```python
from build123d import *

# Parameters (mm, degrees)
SKETCH1_W           = 50.8
SKETCH1_H           = 25.4
BOSS_EXTRUDE1_DEPTH = 5.08
FILLET2_RADIUS      = 2.54
FILLET2_LENGTH      = 25.4
FILLET3_RADIUS      = 2.54
FILLET3_LENGTH      = 25.4
SKETCH2_R           = 2.54
BOSS_EXTRUDE2_DEPTH = 12.7
BOSS_EXTRUDE3_START = 12.7
SKETCH3_R           = 2.54
BOSS_EXTRUDE3_DEPTH = 12.7
SKETCH4_W           = 52.876932696
SKETCH4_H           = 9.818783706
CUT_EXTRUDE1_DEPTH  = 12.7


with BuildPart() as part:
    # Sketch1 → Boss-Extrude1 (new body)
    with BuildSketch(Plane(origin=(0, 0, 0), x_dir=(1, 0, 0), z_dir=(0, 1, 0))):
        Rectangle(SKETCH1_W, SKETCH1_H)
    extrude(amount=BOSS_EXTRUDE1_DEPTH)

    # Fillet2: full round fillet: the end face becomes a half cylinder, R = half its width
    fillet2_face = Plane((-25.4, 2.54, 0), x_dir=(0, 0, -1), z_dir=(-1, 0, 0))  # on the end face: x along it, z out of the body
    fillet2_slab = fillet2_face.offset(-FILLET2_RADIUS / 2) * Box(FILLET2_LENGTH, 2 * FILLET2_RADIUS, FILLET2_RADIUS, mode=Mode.PRIVATE)  # the body's end, R deep
    fillet2_round = Plane((-22.86, 2.54, 0), x_dir=(-1, 0, 0), z_dir=(0, 0, -1)) * Cylinder(FILLET2_RADIUS, FILLET2_LENGTH, mode=Mode.PRIVATE)  # its axis R under the face
    add(fillet2_slab - fillet2_round, mode=Mode.SUBTRACT)

    # Fillet3: full round fillet: the end face becomes a half cylinder, R = half its width
    fillet3_face = Plane((25.4, 2.54, 0), x_dir=(0, 0, 1), z_dir=(1, 0, 0))  # on the end face: x along it, z out of the body
    fillet3_slab = fillet3_face.offset(-FILLET3_RADIUS / 2) * Box(FILLET3_LENGTH, 2 * FILLET3_RADIUS, FILLET3_RADIUS, mode=Mode.PRIVATE)  # the body's end, R deep
    fillet3_round = Plane((22.86, 2.54, 0), x_dir=(1, 0, 0), z_dir=(0, 0, 1)) * Cylinder(FILLET3_RADIUS, FILLET3_LENGTH, mode=Mode.PRIVATE)  # its axis R under the face
    add(fillet3_slab - fillet3_round, mode=Mode.SUBTRACT)

    # Sketch2 → Boss-Extrude2 (add)
    with BuildSketch(Plane(origin=(0, 0, -12.7), x_dir=(-1, 0, 0), z_dir=(0, 0, -1))):
        with Locations((-22.86, 2.54)):
            Circle(SKETCH2_R)
    extrude(amount=BOSS_EXTRUDE2_DEPTH)

    # Sketch3 → Boss-Extrude3 (add)
    with BuildSketch(Plane(origin=(0, 0, -12.7), x_dir=(-1, 0, 0), z_dir=(0, 0, -1)).offset(BOSS_EXTRUDE3_START)):
        with Locations(Location((22.86, 2.54, 0), (0, 0, 90))):
            Circle(SKETCH3_R)
    extrude(amount=-BOSS_EXTRUDE3_DEPTH)

    # Sketch4 → Cut-Extrude1 (cut)
    with BuildSketch(Plane(origin=(0, 0, 0), x_dir=(-1, 0, 0), z_dir=(0, -1, 0))):
        with Locations((0, -12.7)):
            Rectangle(SKETCH4_W, SKETCH4_H)
    extrude(amount=-CUT_EXTRUDE1_DEPTH, mode=Mode.SUBTRACT)


solid = part.part
```
For this review, take the finished solid that the model builds, in its own axes (mm). A direction names the side the tool comes from. Coordinates: 2 decimals unless noted, no trailing zeros. Loops run counter-clockwise (first coordinate to the right, second up) from the corner with the lowest first, then second, coordinate; pieces in that order, holes last.
1. Add section C-C, the plane x = 21.5. Give the boundary of the cut face in (y, z), then the cut area to 3 significant figures.
2. Add section A-A, the plane z = -22.5. Give the boundary of the cut face in (x, y), then the cut area to 3 significant figures.
3. Insertion check: P1, Ø1, axis at y = 1.5, z = -4, coming from the +X side; P2, Ø1, axis at y = 4, z = 0.5, coming from the +X side; P3, Ø12, axis at x = 19, z = -4, coming from the -Y side. Each pin has a flat end and moves straight along its axis. Give the tip position at first contact, or say it passes through.
4. Mouldability with a two-part tool opening along X and no side actions: class faces 3 (the flat face through (0, 5.08, -3)), 4 (the cylindrical face through (-25.113, 3.712, -12.725)) as +X half, -X half, draft (parallel to the pull), parting line (faces both ways), or undercut.
5. Add section B-B, the plane y = 2.54. Give the boundary of the cut face in (x, z).
6. For line 1 (Z direction, x = 4.5, y = 4.5); line 2 (X direction, y = 3.7, z = -15); line 3 (X direction, y = 3.2, z = -22.5), list the stretches that pass through material, from the lowest coordinate up.
7. For faces 1 (the cylindrical face through (25.398, 2.652, -12.26)), 2 (the flat face through (0, 0, -3)), list the 3-axis set-ups (+Z, -Z, +X, -X, +Y, -Y) from which the entire face can be reached by the end or side of a thin tool; tool diameter is ignored.
8. Add section D-D, the plane x = -6. Give the boundary of the cut face in (y, z).
Result:
1. outline: (0, -12.7) - (0.39, -12.7) - (0.39, -25.4) - (4.69, -25.4) - (4.69, -12.7) - (5.08, -12.7) - (5.08, 7.79) - (0, 7.79) - close
1. area: 159 mm2
2. outline: circle Ø5.08 at (-22.86, 2.54); circle Ø5.08 at (22.86, 2.54)
2. area: 40.5 mm2
3. P1: stops at x = 25.34
3. P2: stops at x = 25.21
3. P3: stops at y = 0
4. face 3: draft
4. face 4: undercut
5. outline: (-25.4, -25.4) - (-20.32, -25.4) - (-20.32, -12.7) - (20.32, -12.7) - (20.32, -25.4) - (25.4, -25.4) - (25.4, 7.79) - (-25.4, 7.79) - close
6. line 1: z = -12.7 to 7.79
6. line 2: x = -25.12 to -20.6, 20.6 to 25.12
6. line 3: x = -25.31 to -20.41, 20.41 to 25.31
7. face 1: -Z
7. face 2: +Z, -Z, +X, -X, -Y
8. outline: (0, -12.7) - (5.08, -12.7) - (5.08, 7.79) - (0, 7.79) - close
